For this review, take the finished solid that the model builds, in its own axes (mm). Face numbers are marked on the shaded views. A direction names the side the tool comes from. Coordinates: 2 decimals unless noted, no trailing zeros. Write each loop counter-clockwise with the first axis right and the second up, starting at its lowest first coordinate (ties: lowest second). Pieces come first, ordered by that corner, then holes.
1) We need section A-A on z = -14.5. Write out the cut boundary in (x, y).
2) Insertion check: P1, Ø0.8, axis at x = -0.5, y = -3, coming from the -Z side; P2, Ø2, axis at x = 16.5, y = -1, coming from the -Z side; P3, Ø4, axis at y = 0, z = 31, coming from the -X side. Each pin has a flat end and moves straight along its axis. Give the tip position at first contact, or say it passes through.
3) For the marked faces 1, 2 and 3, list the 3-axis set-ups (+Z, -Z, +X, -X, +Y, -Y) from which the entire face can be reached by the end or side of a thin tool; tool diameter is ignored.
4) We need section C-C on x = -4.5. Write out the cut boundary in (y, z).
5) We need section D-D on z = 15. Write out the cut boundary in (x, y).
6) To check wall thickness, follow line 1 along X through (y, z) = (-0.45, -14.5); line 2 along X through (y, z) = (-0.75, 11); line 3 along X through (y, z) = (-1.1, 5.5). State the ranges of each line that lie inside material, in increasing order.
7) We need section B-B on x = 4.5. Write out the cut boundary in (y, z), then the cut area to 3 significant figures.
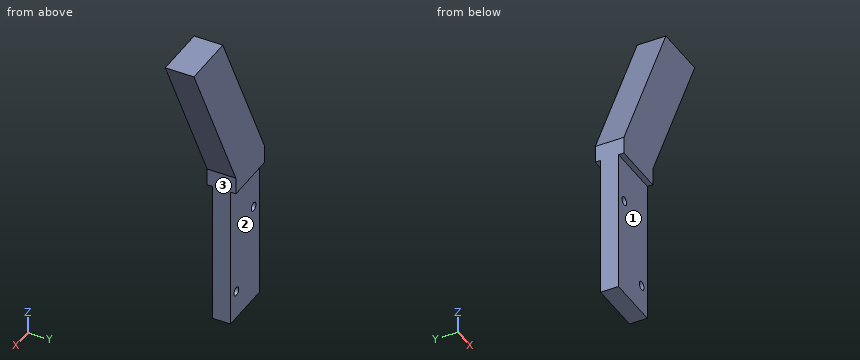
from build123d import *

# Parameters (mm, degrees)
SKETCH1_W           = 15
SKETCH1_H           = 45
SKETCH1_R           = 1.2
BOSS_EXTRUDE1_DEPTH = 2.5
BOSS_EXTRUDE2_DEPTH = 4


with BuildPart() as part:
    # Sketch1 → Boss-Extrude1 (new body, symmetric)
    with BuildSketch(Plane(origin=(0, 0, 0), x_dir=(1, 0, 0), z_dir=(0, 1, 0))):
        Rectangle(SKETCH1_W, SKETCH1_H)
        with Locations((-4.5, -5.5)):
            Circle(SKETCH1_R, mode=Mode.SUBTRACT)
        with Locations((4.5, 14.5)):
            Circle(SKETCH1_R, mode=Mode.SUBTRACT)
    extrude(amount=BOSS_EXTRUDE1_DEPTH, both=True)

    # Sketch4 → Boss-Extrude2 (add, symmetric)
    with BuildSketch(Plane(origin=(0, 0, 0), x_dir=(1, 0, 0), z_dir=(0, 1, 0))):
        Polygon((-7.5, -17.715662228), (-7.5, -22.5), (14.294494718, -67.5), (29.294494718, -67.5), (7.5, -22.5), (7.5, -17.715662228), align=None)
    extrude(amount=BOSS_EXTRUDE2_DEPTH, both=True)


solid = part.part
Result:
1. outline: (-7.5, -2.5) - (3.3, -2.5) - (3.3, 2.5) - (-7.5, 2.5) - close; (5.7, -2.5) - (7.5, -2.5) - (7.5, 2.5) - (5.7, 2.5) - close
2. P1: stops at z = 17.72
2. P2: stops at z = 39.02
2. P3: stops at x = -4.35
3. face 1: -Z, +X, -X, -Y
3. face 2: -Z, +X, -X, +Y
3. face 3: -Z, +X, +Y, -Y
4. outline: (-4, 17.72) - (-2.5, 17.72) - (-2.5, 6.7) - (2.5, 6.7) - (2.5, 17.72) - (4, 17.72) - (4, 28.69) - (-4, 28.69) - close; (-2.5, -22.5) - (2.5, -22.5) - (2.5, 4.3) - (-2.5, 4.3) - close
5. outline: (-7.5, -2.5) - (7.5, -2.5) - (7.5, 2.5) - (-7.5, 2.5) - close
6. line 1: x = -7.5 to 3.3, 5.7 to 7.5
6. line 2: x = -7.5 to 7.5
6. line 3: x = -7.5 to -5.7, -3.3 to 7.5
7. outline: (-4, 17.72) - (-2.5, 17.72) - (-2.5, -13.3) - (2.5, -13.3) - (2.5, 17.72) - (4, 17.72) - (4, 47.28) - (-4, 47.28) - close; (-2.5, -22.5) - (2.5, -22.5) - (2.5, -15.7) - (-2.5, -15.7) - close
7. area: 426 mm2
